The listing builds one solid part. Answer for the finished solid, in the listing's coordinates (mm). Give positions to 0.01 mm unless a question says otherwise; leave off trailing zeros. Order: outer loops, then holes, each group sorted by start corner. A loop starts at its lowest first (then second) coordinate and runs counter-clockwise, first axis right, second up. Notation, with made-up numbers: (2.25, 39) - (21.25, 39) arc R24 cw to (21.25, 51) - close; hole circle Ø8 at (51, 46). An arc over 180 degrees is marked (long way). Answer as CSV lines item,"result". Start each with the question number.
1. Flat-ended cylindrical pins translate along their axes: pin 1 (3 mm diameter, centred on x = -4, y = -4.5, fed in from +Z); pin 2 (5 mm diameter, centred on x = -1, y = 8, fed in from +Z); pin 3 (13 mm diameter, centred on y = -6.5, z = -14.5, fed in from -X). Find the tip coordinate at first contact, or state that the pin passes through.
2. Section B-B on y = -5 is taken. Give the vertices of the cut face in (x, z), and give its area (3 significant figures).
3. Consider line 1 along Z through (x, y) = (-5.25, 11.5); line 2 along Z through (x, y) = (0, 16.5); line 3 along Y through (x, z) = (-1, 15). Determine where each line is inside the solid, lowest interval first. Write a range as [from, to].
4. Section A-A on z = 0 is taken. Give the vertices of the cut face in (x, y), and give its area (3 significant figures).
5. Section C-C on x = 0 is taken. Give the vertices of the cut face in (y, z), and give its area (3 significant figures).
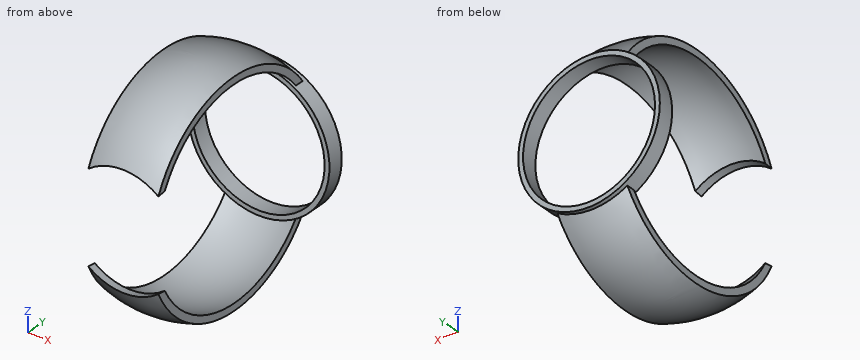
Autodesk Inventor part; units mm, degrees
ref_plane "XY Plane" through (0, 0, 0) normal (0, 0, 1) x (1, 0, 0)
sketch "Sketch1" plane through (0, 0, 0) normal (0, 1, 0) x (-1, 0, 0)
  circle A0 centre (0, 0) radius 21.59
  line L0 (0, -21.59) -> (0, 21.59)
  dimension "d0" = 43.18
revolve "Revolution1" add sketch "Sketch1" angle 360 about axis through (0, 0, -21.59) along (0, 0, 1)
sketch "Sketch2" plane through (0, 0, 0) normal (0, 1, 0) x (-1, 0, 0)
  line L0 (-6.604, -23.7777) -> (-21.7081, -23.7777)
  line L1 (-21.7081, -23.7777) -> (-21.7081, 23.9273)
  line L2 (-21.7081, 23.9273) -> (-6.604, 23.9273)
  line L3 (-6.604, 23.9273) -> (-6.604, -23.7777)
  line L4 (6.604, 26.32) -> (23.3531, 26.32)
  line L5 (23.3531, 26.32) -> (23.3531, -25.5723)
  line L6 (23.3531, -25.5723) -> (6.604, -25.5723)
  line L7 (6.604, -25.5723) -> (6.604, 26.32)
  point P0 (0, 0)
  dimension "d2" = 6.604
  dimension "d3" = 6.604
extrude "Extrusion1" cut sketch "Sketch2" along normal mid plane 50.8
sketch "Sketch3" plane through (0, 0, 0) normal (0, 1, 0) x (-1, 0, 0)
  circle A0 centre (0, 0) radius 12.446
  dimension "d6" = 24.892
extrude "Extrusion2" cut sketch "Sketch3" along normal blind 47.625 and the other way blind 22.2377 draft -5
sketch "Sketch4" plane through (0, 0, 0) normal (0, 1, 0) x (-1, 0, 0)
  circle A0 centre (0, 0) radius 20.32
  line L0 (20.32, 0) -> (-20.32, 0)
  dimension "d11" = 40.64
revolve "Revolution2" cut sketch "Sketch4" angle 360 about axis through (-20.32, 0, 0) along (1, 0, 0)
sketch "Sketch5" plane through (0, 0, 0) normal (0, 1, 0) x (-1, 0, 0)
  circle A0 centre (0, 0) radius 13.3548
  circle A1 centre (0, 0) radius 12.446
extrude "Extrusion3" add sketch "Sketch5" along normal blind 17.78
sketch "Sketch6" plane through (0, 0, 0) normal (0, 1, 0) x (-1, 0, 0)
  circle A0 centre (0, 0) radius 12.446
  circle A1 centre (0, 0) radius 12.446
  circle A2 centre (0, 0) radius 13.3548
extrude "Extrusion4" cut sketch "Sketch6" along normal blind 14.732
properties part number "mid_panel"
Checks:
1,pin 1,"stops at z = 21.11"
1,pin 2,"stops at z = 20.86"
1,pin 3,"stops at x = -6.6"
2,outline,"(-6.6, -19.94) arc R21 ccw to (6.6, -19.94) - (6.6, -18.56) arc R19.7 cw to (-6.6, -18.56) - close; (-6.6, 18.56) arc R19.7 cw to (6.6, 18.56) - (6.6, 19.94) arc R21 ccw to (-6.6, 19.94) - close"
2,area,"35.2 mm²"
3,line 1,"z = [-17.5, -15.91], [15.91, 17.5]"
3,line 2,"z = [-13.92, -12.45], [12.45, 13.92]"
3,line 3,"y = [-15.5, -13.67], [13.67, 15.5]"
4,outline,"(-13.35, 14.73) - (-12.45, 14.73) - (-12.45, 17.78) - (-13.35, 17.78) - close; (12.45, 14.73) - (13.35, 14.73) - (13.35, 17.78) - (12.45, 17.78) - close"
4,area,"5.54 mm²"
5,outline,"(-18.69, -10.81) arc R21.59 ccw to (16.96, -13.35) - (17.78, -13.35) - (17.78, -12.45) - (14.73, -12.45) - (14.73, -13.35) - (15.32, -13.35) arc R20.32 cw to (-17.12, -10.95) - close; (-18.69, 10.81) - (-17.12, 10.95) arc R20.32 cw to (15.32, 13.35) - (14.73, 13.35) - (14.73, 12.45) - (17.78, 12.45) - (17.78, 13.35) - (16.96, 13.35) arc R21.59 ccw to start"
5,area,"107 mm²"
